Source: CAD feature listing. Evaluate the final solid. Frame: model axes, mm. Give positions to 0.01 mm unless a question says otherwise; leave off trailing zeros. Order: outer loops, then holes, each group sorted by start corner. A loop starts at its lowest first (then second) coordinate and runs counter-clockwise, first axis right, second up. Notation, with made-up numbers: M 70,73 L 76,73 A34 cw 76,104 Z; hole C 80.5,-36.5 d8. An arc over 180 degrees is marked long. Use CSV: the item, a comma, the result in double quotes. Start each with the question number.
Item 1: Section query A-A on z = -7. Return loops of the section in (x, y).
Item 2: Ray query, probe 1 along Z at (x, y) = (65.5, 2.65); probe 2 along Z at (x, y) = (56.5, 1.1). Return the intervals inside material, ascending. Write a range as from..to.
Item 3: First-contact query: pin 1 (2 mm diameter, centred on x = 53, y = 1, fed in from -Z); pin 2 (1.5 mm diameter, centred on y = 1, z = -3.5, fed in from +X); pin 3 (2 mm diameter, centred on x = 20.5, y = 1.5, fed in from +Z); pin 4 (12 mm diameter, centred on x = 122, z = -11, fed in from -Y). Flat tips, straight axial feed; report the tip coordinate or a pass-through.
Item 4: Section query B-B on x = 50.5. Return loops of the section in (y, z).
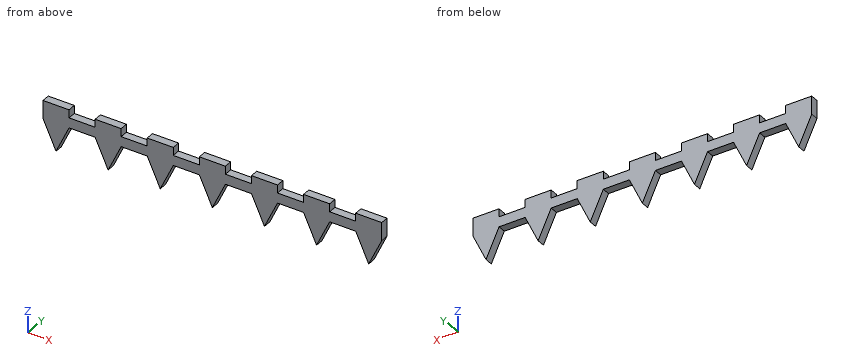
from build123d import *

# Parameters (mm, degrees)
F0_W     = 13
F0_H     = 4
F1_DEPTH = 5
F2_DEPTH = 9
F4_DEPTH = 4


with BuildPart() as f1:
    # F0 (on Top) → F1 (new body)
    with BuildSketch(Plane.XY):
        with Locations((6.5, 2)):
            Rectangle(F0_W, F0_H)
        with Locations((19.5, 2)):
            Rectangle(F0_W, F0_H)
        with Locations((32.5, 2)):
            Rectangle(F0_W, F0_H)
        with Locations((45.5, 2)):
            Rectangle(F0_W, F0_H)
        with Locations((58.5, 2)):
            Rectangle(F0_W, F0_H)
        with Locations((71.5, 2)):
            Rectangle(F0_W, F0_H)
        with Locations((84.5, 2)):
            Rectangle(F0_W, F0_H)
        with Locations((97.5, 2)):
            Rectangle(F0_W, F0_H)
        with Locations((110.5, 2)):
            Rectangle(F0_W, F0_H)
        with Locations((123.5, 2)):
            Rectangle(F0_W, F0_H)
        with Locations((136.5, 2)):
            Rectangle(F0_W, F0_H)
        with Locations((149.5, 2)):
            Rectangle(F0_W, F0_H)
        with Locations((162.5, 2)):
            Rectangle(F0_W, F0_H)
    extrude(amount=F1_DEPTH)

    # F0 (on Top) → F2 (join)
    with BuildSketch(Plane.XY):
        with Locations((6.5, 2)):
            Rectangle(F0_W, F0_H)
        with Locations((32.5, 2)):
            Rectangle(F0_W, F0_H)
        with Locations((58.5, 2)):
            Rectangle(F0_W, F0_H)
        with Locations((84.5, 2)):
            Rectangle(F0_W, F0_H)
        with Locations((110.5, 2)):
            Rectangle(F0_W, F0_H)
        with Locations((136.5, 2)):
            Rectangle(F0_W, F0_H)
        with Locations((162.5, 2)):
            Rectangle(F0_W, F0_H)
    extrude(amount=F2_DEPTH)

    # F3 (on face) → F4 (join)
    with BuildSketch(Plane.XZ):
        Polygon((13, 0), (0, 0), (6.5, -14), align=None)
        Polygon((39, 0), (26, 0), (32.5, -14), align=None)
        Polygon((65, 0), (52, 0), (58.5, -14), align=None)
        Polygon((91, 0), (78, 0), (84.5, -14), align=None)
        Polygon((117, 0), (104, 0), (110.5, -14), align=None)
        Polygon((143, 0), (130, 0), (136.5, -14), align=None)
        Polygon((162.5, 0), (156, 0), (162.5, -14), align=None)
        Polygon((162.5, 0), (162.5, -14), (169, 0), align=None)
    extrude(amount=-F4_DEPTH)


solid = f1.part
Verdict:
1,outline,"M 3.25,0 L 9.75,0 L 9.75,4 L 3.25,4 Z; M 29.25,0 L 35.75,0 L 35.75,4 L 29.25,4 Z; M 55.25,0 L 61.75,0 L 61.75,4 L 55.25,4 Z; M 81.25,0 L 87.75,0 L 87.75,4 L 81.25,4 Z; M 107.25,0 L 113.75,0 L 113.75,4 L 107.25,4 Z; M 133.25,0 L 139.75,0 L 139.75,4 L 133.25,4 Z; M 159.25,0 L 165.75,0 L 165.75,4 L 159.25,4 Z"
2,probe 1,"0..5"
2,probe 2,"-9.69..9"
3,pin 1,"z = -4.31"
3,pin 2,"x = 167.72"
3,pin 3,"z = 5"
3,pin 4,"through"
4,outline,"M 0,0 L 4,0 L 4,5 L 0,5 Z"
